Could you check a few things on this model? Use its own coordinates, in mm. Face numbers are marked on the shaded views. Give positions to 0.01 mm unless a question says otherwise; leave off trailing zeros. Write each question's results on one line, items separated by ' | '.
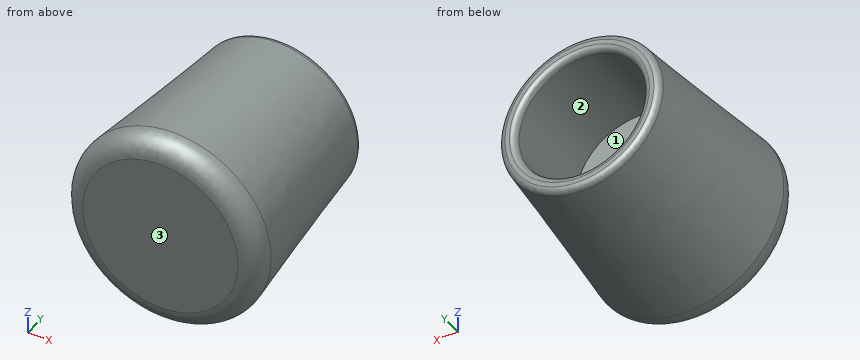
```python
from build123d import *

# Parameters (mm, degrees)
SKETCH2_R          = 8.128
CUT_EXTRUDE1_DEPTH = 12.7
FILLET1_R          = 2.54
FILLET2_R          = 0.762


with BuildPart() as part:
    # Loft1: read off the stored shape, not the designer's step
    # Loft1: loft between two sections, ruled curve by curve
    loft1_from = [
        Edge.make_bspline([(-6.387278158, 25.4, 7.901156734), (-22.189591626, 25.4, -4.873399581), (-9.41503531, 25.4, -20.675713049), (6.387278158, 25.4, -7.901156734), (22.189591626, 25.4, 4.873399581), (9.41503531, 25.4, 20.675713049), (-6.387278158, 25.4, 7.901156734)], [0, 0, 0, 0, 0.5, 0.5, 0.5, 1, 1, 1, 1], 3, [1, 0.333333333, 0.333333333, 1, 0.333333333, 0.333333333, 1]),
    ]
    loft1_to = [
        Edge.make_bspline([(-5.094992756, 0, 11.633187388), (-28.361367533, 0, 1.443201876), (-18.17138202, 0, -21.823172901), (5.094992756, 0, -11.633187388), (28.361367533, 0, -1.443201876), (18.17138202, 0, 21.823172901), (-5.094992756, 0, 11.633187388)], [0, 0, 0, 0, 0.5, 0.5, 0.5, 1, 1, 1, 1], 3, [1, 0.333333333, 0.333333333, 1, 0.333333333, 0.333333333, 1]),
    ]
    loft1 = Solid(Shell([*[Face.make_surface_from_curves(loft1_from[k], loft1_to[k]) for k in range(1)], Face(Wire(loft1_from)), Face(Wire(loft1_to))]))
    add(loft1)

    # Sketch2 → Cut-Extrude1 (cut)
    with BuildSketch(Plane(origin=(0, 25.4, 0), x_dir=(1, 0, 0), z_dir=(0, 1, 0))):
        with Locations(Location((0, 0, 0), (0, 0, 270))):
            Circle(SKETCH2_R)
    extrude(amount=-CUT_EXTRUDE1_DEPTH, mode=Mode.SUBTRACT)

    # Fillet1
    fillet1_edges = [part.edges().sort_by_distance(p)[0] for p in [
        (5.094992756, 0, -11.633187388),
    ]]
    fillet(fillet1_edges, radius=FILLET1_R)

    # Fillet2
    fillet2_edges = [part.edges().sort_by_distance(p)[0] for p in [
        (6.387278158, 25.4, -7.901156734),
        (0, 25.4, -8.128),
    ]]
    fillet(fillet2_edges, radius=FILLET2_R)


solid = part.part
```
Q1. I need wall thicknesses on line 1 along Y through (x, z) = (5, 1.75); line 2 along Z through (x, y) = (7.25, 22); line 3 along X through (y, z) = (19.25, 0). Which ranges of each line are inside material? Lowest first, please.
Here are the results:
line 1: y = 0 to 12.7 | line 2: z = -7.53 to -3.67, 3.67 to 7.53 | line 3: x = -10.7 to -8.13, 8.13 to 10.7
Q2. I'm going to push flat-ended pins straight in: pin 1 Ø2 at (x, y) = (-2, 10.5) entering from -Z; pin 2 Ø8 at (y, z) = (9.5, 2.5) entering from -X; pin 3 Ø1.5 at (y, z) = (17.5, -9) entering from +X. Where does each tip first touch, or does it pass through?
Here are the results:
pin 1: stops at z = -11.56 | pin 2: stops at x = -12.02 | pin 3: stops at x = 7.07
Q3. Thinking about a two-plate mould opening in Z: for the marked faces 1, 2 and 3, which applies, +Z half, -Z half, draft (parallel to the pull), parting line (faces both ways), or undercut?
Here are the results:
face 1: undercut | face 2: undercut | face 3: draft
